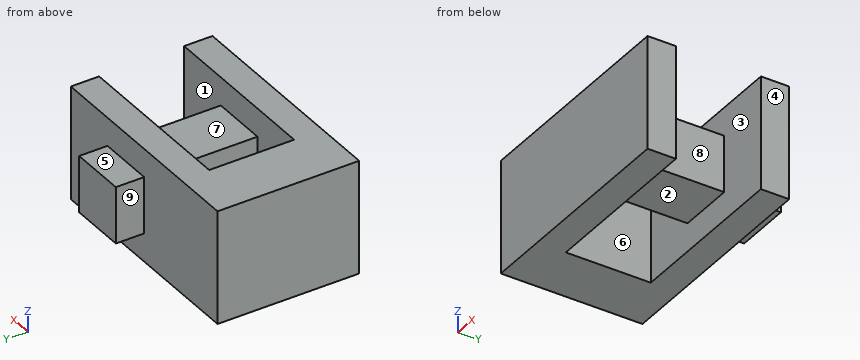
from build123d import *

# Parameters (mm, degrees)
BOSS_EXTRUDE1_DEPTH             = 20
SKETCH2_W                       = 10
SKETCH2_H                       = 10
BOSS_EXTRUDE2_DEPTH             = 5
BOSS_EXTRUDE2_DIRECTION_2_REACH = 53.235


with BuildPart() as part:
    # Sketch1 → Boss-Extrude1 (new body)
    with BuildSketch(Plane.XY):
        Polygon((0, 0), (40, 0), (40, 5), (10, 5), (10, 20), (40, 20), (40, 25), (0, 25), align=None)
    extrude(amount=BOSS_EXTRUDE1_DEPTH)

    # Sketch2 → Boss-Extrude2 (add)
    with BuildSketch(Plane(origin=(0, 25, 0), x_dir=(1, 0, 0), z_dir=(0, 1, 0))):
        with Locations((25, -10)):
            Rectangle(SKETCH2_W, SKETCH2_H)
    extrude(amount=BOSS_EXTRUDE2_DEPTH)

    # Sketch2 → Boss-Extrude2 direction 2 (add, up to next)
    with BuildSketch(Plane(origin=(0, 25, 0), x_dir=(1, 0, 0), z_dir=(0, 1, 0)), mode=Mode.PRIVATE) as boss_extrude2_direction_2_sk1:
        with Locations((25, -10)):
            Rectangle(SKETCH2_W, SKETCH2_H)
    boss_extrude2_direction_2_tool1 = extrude(boss_extrude2_direction_2_sk1.sketch, amount=-BOSS_EXTRUDE2_DIRECTION_2_REACH, mode=Mode.PRIVATE) - part.part
    add(boss_extrude2_direction_2_tool1.solids().sort_by_distance((25, 25, 10))[0])


solid = part.part
Read the model definition and answer for the solid it produces. Units are mm, in the model's axes. Face numbers are marked on the shaded views. A direction names the side the tool comes from. Round coordinates to 2 decimals unless told otherwise and drop trailing zeros. Order: outer loops, then holes, each group sorted by start corner. A loop starts at its lowest first (then second) coordinate and runs counter-clockwise, first axis right, second up.
1) The part is cut by section B-B on z = 6.5. Write down the section's boundary in (x, y).
2) The part is cut by section A-A on x = 16.5. Write down the section's boundary in (y, z).
3) Straight lines are drawn through the part: L1, parallel to X at y = 13.25, z = 12.75; L2, parallel to Y at x = 30.5, z = 15.25; L3, parallel to Z at x = 20.5, y = 7.25. For each, find the intervals that lie inside material, in ascending order.
4) For the marked faces 5, 6, 7, 8 and 9, determine the directions among +Z, -Z, +X, -X, +Y, -Y from which every point of the face is accessible in a straight line to the end or side of a thin tool.
5) The mould has two halves that part along X. Classify the marked faces 1, 2, 3 and 4: released by +X, released by -X, zero draft, split by the parting line, or undercut.
6) The part is cut by section C-C on y = 10.25. Write down the section's boundary in (x, z), plus the area to 3 significant figures.
7) The part is cut by section D-D on x = 21. Write down the section's boundary in (y, z).
8) Flat-ended cylindrical pins translate along their axes: pin 1 (10 mm diameter, centred on x = 26.5, y = 13, fed in from +Z); pin 2 (7.5 mm diameter, centred on y = 10.5, z = 10.5, fed in from +X); pin 3 (4 mm diameter, centred on y = 27.5, z = 9.5, fed in from -X). Find the tip coordinate at first contact, or state that the pin passes through.
Resolved:
1. outline: (0, 0) - (40, 0) - (40, 5) - (30, 5) - (30, 20) - (40, 20) - (40, 25) - (30, 25) - (30, 30) - (20, 30) - (20, 25) - (0, 25) - close; hole (10, 5) - (20, 5) - (20, 20) - (10, 20) - close
2. outline: (0, 0) - (5, 0) - (5, 20) - (0, 20) - close; (20, 0) - (25, 0) - (25, 20) - (20, 20) - close
3. L1: x = 0 to 10, 20 to 30
3. L2: y = 0 to 5, 20 to 25
3. L3: z = 5 to 15
4. face 5: +Z, +X, -X, +Y
4. face 6: +Z, -Z
4. face 7: +Z, +X
4. face 8: +Z, -Z, +X
4. face 9: +Z, -Z, -X, +Y
5. face 1: undercut
5. face 2: zero draft
5. face 3: undercut
5. face 4: released by +X
6. outline: (0, 0) - (10, 0) - (10, 20) - (0, 20) - close; (20, 5) - (30, 5) - (30, 15) - (20, 15) - close
6. area: 300 mm2
7. outline: (0, 0) - (5, 0) - (5, 5) - (20, 5) - (20, 0) - (25, 0) - (25, 5) - (30, 5) - (30, 15) - (25, 15) - (25, 20) - (20, 20) - (20, 15) - (5, 15) - (5, 20) - (0, 20) - close
8. pin 1: stops at z = 15
8. pin 2: stops at x = 30
8. pin 3: stops at x = 20
